Work out the finished part from the listing and answer in its coordinate system (mm). Give positions to 0.01 mm unless a question says otherwise; leave off trailing zeros. Order: outer loops, then holes, each group sorted by start corner. A loop starts at its lowest first (then second) coordinate and runs counter-clockwise, first axis right, second up. Notation, with made-up numbers: (-5.5, 79) - (3.5, 79) arc R35 cw to (3.5, 116) - close; hole circle Ø7 at (61, 1.25). An arc over 180 degrees is marked (long way). Write each question's results on one line, items separated by ' | '.
Autodesk Inventor part; units mm, degrees
ref_plane "Work Plane1" through (-24.15, -24.15, 49.8) normal (0, 0, 1) x (1, 0, 0)
ref_plane "YZ Plane" through (0, 0, 0) normal (1, 0, 0) x (0, 1, 0)
ref_plane "XZ Plane" through (0, 0, 0) normal (0, 1, 0) x (-1, 0, 0)
sketch "Sketch1" plane through (0, 0, 0) normal (0, 0, 1) x (1, 0, 0)
  circle A0 centre (-21.9, -21.9) radius 1.875
  circle A1 centre (21.9, 21.9) radius 1.875
  circle A2 centre (21.9, -21.9) radius 1.875
  circle A3 centre (-21.9, 21.9) radius 1.875
  circle A4 centre (14.4, 20.8) radius 2.0734
  circle A5 centre (-14.4, -20.8) radius 2.0734
  circle A6 centre (14.4, -20.8) radius 2.0734
  circle A7 centre (20.8, -14.4) radius 2.0734
  line L0 (-17.05, 17.05) -> (-17.05, -17.05)
  line L1 (17.05, 17.05) -> (-17.05, 17.05)
  line L2 (17.05, -17.05) -> (17.05, 17.05)
  line L3 (-17.05, -17.05) -> (17.05, -17.05)
  circle A8 centre (20.8, 14.4) radius 2.0734
  circle A9 centre (-14.4, 20.8) radius 2.0734
  circle A10 centre (-20.8, -14.4) radius 2.0734
  circle A11 centre (-20.8, 14.4) radius 2.0734
  line L4 (-22.9, 24.875) -> (22.9, 24.875)
  arc A12 (-22.9, 24.875) -> (-24.875, 22.9) centre (-22.9, 22.9) ccw
  line L5 (-24.875, -22.9) -> (-24.875, 22.9)
  arc A13 (-24.875, -22.9) -> (-22.9, -24.875) centre (-22.9, -22.9) ccw
  line L6 (22.9, -24.875) -> (-22.9, -24.875)
  arc A14 (22.9, -24.875) -> (24.875, -22.9) centre (22.9, -22.9) ccw
  line L7 (24.875, 22.9) -> (24.875, -22.9)
  arc A15 (24.875, 22.9) -> (22.9, 24.875) centre (22.9, 22.9) ccw
  point P0 (0, 0)
ref_plane "Work Plane1" through (-24.15, -24.15, 49.8) normal (0, 0, 1) x (1, 0, 0)
extrude "Extrusion1" add sketch "Sketch1" along normal blind 1.5 from surface at 49.8 contours A0 | A1 | A2 | A3 | L1 L2 L3 L0 | L4 A15 L7 A14 L6 A13 L5 A12
sketch "Sketch2" plane through (-22.9, -24.875, 51.3) normal (0, 0, 1) x (1, 0, 0)
  arc A0 (-1.975, 1.975) -> (0, 0) centre (0, 1.975) ccw
  line L0 (45.8, 0) -> (0, 0)
  arc A1 (45.8, 0) -> (47.775, 1.975) centre (45.8, 1.975) ccw
  line L1 (47.775, 47.775) -> (47.775, 1.975)
  arc A2 (47.775, 47.775) -> (45.8, 49.75) centre (45.8, 47.775) ccw
  line L2 (0, 49.75) -> (45.8, 49.75)
  arc A3 (0, 49.75) -> (-1.975, 47.775) centre (0, 47.775) ccw
  line L3 (-1.975, 1.975) -> (-1.975, 47.775)
  circle A4 centre (2.1, 39.275) radius 2.0734
  circle A5 centre (2.1, 10.475) radius 2.0734
  circle A6 centre (8.5, 45.675) radius 2.0734
  circle A7 centre (43.7, 39.275) radius 2.0734
  circle A8 centre (43.7, 10.475) radius 2.0734
  circle A9 centre (37.3, 4.075) radius 2.0734
  circle A10 centre (8.5, 4.075) radius 2.0734
  circle A11 centre (37.3, 45.675) radius 2.0734
  arc A12 (48.625, 47.775) -> (45.8, 50.6) centre (45.8, 47.775) ccw
  line L4 (48.625, 47.775) -> (48.625, 1.975)
  arc A13 (45.8, -0.85) -> (48.625, 1.975) centre (45.8, 1.975) ccw
  line L5 (45.8, -0.85) -> (0, -0.85)
  arc A14 (-2.825, 1.975) -> (0, -0.85) centre (0, 1.975) ccw
  line L6 (-2.825, 1.975) -> (-2.825, 47.775)
  arc A15 (0, 50.6) -> (-2.825, 47.775) centre (0, 47.775) ccw
  line L7 (0, 50.6) -> (45.8, 50.6)
  line L8 (47.775, 1.975) -> (45.8, 1.975)
  line L9 (45.8, 1.975) -> (45.8, -0.85)
  line L10 (45.8, -0.85) -> (47.775, -0.85)
  line L11 (47.775, -0.85) -> (47.775, 1.975)
  line L12 (-1.975, 1.975) -> (0, 1.975)
  line L13 (0, 1.975) -> (0, -0.85)
  line L14 (0, -0.85) -> (-1.975, -0.85)
  line L15 (-1.975, -0.85) -> (-1.975, 1.975)
  line L16 (-1.975, 47.775) -> (0, 47.775)
  line L17 (0, 47.775) -> (0, 50.6)
  line L18 (0, 50.6) -> (-1.975, 50.6)
  line L19 (-1.975, 50.6) -> (-1.975, 47.775)
  line L20 (47.775, 47.775) -> (45.8, 47.775)
  line L21 (45.8, 47.775) -> (45.8, 50.6)
  line L22 (45.8, 50.6) -> (47.775, 50.6)
  line L23 (47.775, 50.6) -> (47.775, 47.775)
  point P0 (22.9, 24.875)
  dimension "d2" = 0.85
extrude "Extrusion2" add sketch "Sketch2" against normal blind 1.5 contours A0 L13 A14 L15 | L0 L9 L5 L13 | L19 A15 L17 A3 | A14 L14 L15 | A1 L11 A13 L9 | L17 L7 L21 L2 | L19 L18 A15 | A13 L11 L10 | L21 A12 L23 A2 | L22 L23 A12
chamfer "Chamfer1" distance 1.5 angle 45 2 edges at (0, 25.725, 51.3) (0, -25.725, 51.3)
properties part number "Panel Top 1x1"
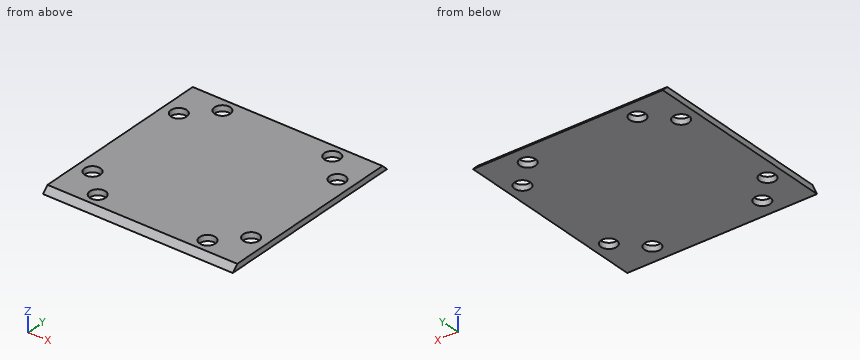
1. A cutting plane is placed at A-A, the plane y = -14.4. Write down the section's boundary in (x, z) (3 decimals).
Answer list:
outline: (-24.875, 49.8) - (-22.873, 49.8) - (-22.873, 51.3) - (-24.875, 51.3) - close; (-18.727, 49.8) - (18.727, 49.8) - (18.727, 51.3) - (-18.727, 51.3) - close; (22.873, 49.8) - (24.875, 49.8) - (24.875, 51.3) - (22.873, 51.3) - close
2. Straight lines are drawn through the part: line 1 (X direction, y = -14.5, z = 51.2) (3 decimals); line 2 (X direction, y = 21, z = 51.25) (3 decimals); line 3 (Y direction, x = -16, z = 50.7). For each, find the intervals that lie inside material, in ascending order. Write a range as [from, to].
Answer list:
line 1: [-24.875, -22.871], [-18.729, 18.729], [22.871, 24.875] | line 2: [-24.875, -16.464], [-12.336, 12.336], [16.464, 24.875] | line 3: [-24.83, -22.12], [-19.48, 19.48], [22.12, 24.83]
3. A cutting plane is placed at B-B, the plane x = 14.4. State how many separate pieces and enclosed holes the cut face has, then the cut area to 3 significant figures.
Answer list:
separate pieces: 3 | enclosed holes: 0 | area: 62.5 mm^2
